Design review of the part built by this model. Coordinates are the model's own, in mm. Face numbers are marked on the shaded views. Give positions to 0.01 mm unless a question says otherwise; leave off trailing zeros. Write each loop counter-clockwise with the first axis right and the second up, starting at its lowest first coordinate (ties: lowest second). Pieces come first, ordered by that corner, then holes. Notation, with made-up numbers: (-32.75, 86.5) -> (-27.75, 86.5) arc R15 cw to (-27.75, 100.5) -> close; hole circle Ø8 at (2.25, -40). An arc over 180 degrees is marked (long way). Use CSV: the item, a comma, the result in double quotes.
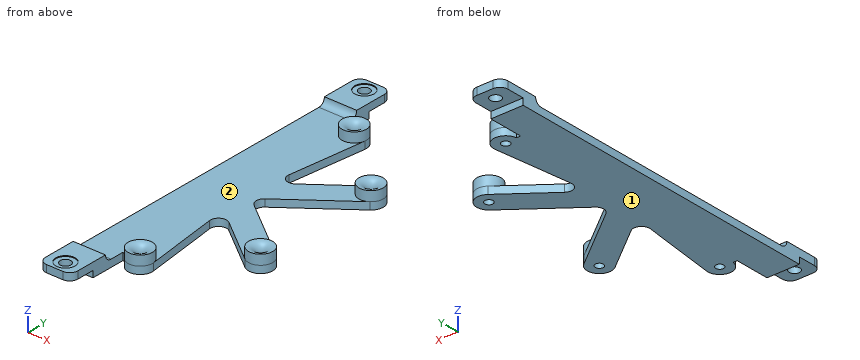
```python
from build123d import *

# Parameters (mm, degrees)
SKETCH_1_W                   = 20
SKETCH_1_H                   = 232
EXTRUDE_1_DEPTH              = 4.5
EXTRUDE_3_DEPTH              = 4.5
FILLET_2_R                   = 4.999999999999999
HOLE_WIZARD_M6_1_D           = 5
FILLET_4_R                   = 4.999999999999999
EXTRUDE_START                = 4
EXTRUDE_4_DEPTH              = 4
SKETCH_9_W                   = 319.0213755361433
SKETCH_9_H                   = 251.11270465686212
CUT_EXTRUDE_1_DEPTH          = 4
FILLET_5_R                   = 4
HOLE_WIZARD_M6_2_D           = 6.6
HOLE_WIZARD_M6_2_CBORE_D     = 12
HOLE_WIZARD_M6_2_CBORE_DEPTH = 0.5
EXTRUDE_START_2              = 6
SKETCH_13_R                  = 2.4999999999999987
SKETCH_13_R_2                = 2.499999999999995
EXTRUDE_5_DEPTH              = 6
FILLET_6_R                   = 5


# Some blends are built 0.0001 mm under size
with BuildPart() as part:
    # 草图1 → 凸台-拉伸1 (new body)
    with BuildSketch(Plane.XY):
        Rectangle(SKETCH_1_W, SKETCH_1_H)
    extrude(amount=EXTRUDE_1_DEPTH)

    # 草图4 → 凸台-拉伸3 (add)
    with BuildSketch(Plane.XY.offset(4.5)):
        with BuildLine():
            Line((67.04532411447143, -34.03426209975627), (22.3753551085413, -8.9e-16))
            Line((22.375355108541303, -2.66e-15), (67.04532411447141, 34.0342620997563))
            ThreePointArc((67.04532411447141, 34.03426209975629), (68.46573790024371, 44.54532411447144), (57.954675885528566, 45.96573790024377))
            Line((57.954675885528566, 45.96573790024377), (19.735945661830147, 16.846705348854464))
            Line((19.73594566183015, 16.846705348854464), (27.438333999755184, 76.54021496777352))
            ThreePointArc((27.438333999755184, 76.54021496777352), (20.959785032226467, 84.9383339997552), (12.561666000244795, 78.45978503222648))
            Line((12.561666000244797, 78.45978503222648), (10.000000000000002, 78.45978503222645))
            Line((10.000000000000002, 78.45978503222645), (9.999999999999897, 58.60687353032759))
            Line((9.999999999999785, 58.606873530327604), (2.561666000244813, 0.9597850322264776))
            ThreePointArc((2.5616660002448137, 0.9597850322264744), (2.5000000000000036, -1.321e-14), (2.561666000244818, -0.9597850322265004))
            Line((2.561666000244811, -0.959785032226501), (9.999999999999945, -58.606873530328755))
            Line((9.999999999999973, -58.606873530328755), (10.000000000000002, -78.45978503222648))
            Line((10.000000000000002, -78.45978503222648), (12.561666000244813, -78.45978503222648))
            ThreePointArc((12.561666000244813, -78.45978503222648), (20.95978503222648, -84.9383339997552), (27.43833399975519, -76.54021496777352))
            Line((27.438333999755194, -76.54021496777352), (19.735945661830147, -16.846705348854485))
            Line((19.735945661830144, -16.84670534885448), (57.95467588552857, -45.96573790024377))
            ThreePointArc((57.95467588552857, -45.96573790024377), (68.46573790024374, -44.54532411447145), (67.04532411447143, -34.034262099756276))
        make_face()
    extrude(amount=-EXTRUDE_3_DEPTH)

    # 圆角2
    fillet_2_edges = [part.edges().sort_by_distance(p)[0] for p in [
        (19.735945661830144, -16.846705348854485, 2.25),
        (22.3753551085413, -1.78e-15, 2.25),
        (19.73594566183015, 16.846705348854464, 2.25),
    ]]
    fillet(fillet_2_edges, radius=FILLET_2_R)

    # Hole Wizard M6 _1 (through all)
    with Locations(Plane.XY.offset(4.5)):
        with Locations((20, 77.5), (62.5, 40), (20, -77.5), (62.5, -40)):
            Hole(HOLE_WIZARD_M6_1_D / 2)

    # 圆角4
    fillet_4_edges = [part.edges().sort_by_distance(p)[0] for p in [
        (10.000000000000002, -116.00000000000001, 2.25),
        (-9.999999999999998, -116.00000000000001, 2.25),
        (-9.999999999999998, 115.99999999999999, 2.25),
        (10.000000000000002, 115.99999999999999, 2.25),
    ]]
    fillet(fillet_4_edges, radius=FILLET_4_R)

    # 草图8 → 凸台-拉伸4 (add)
    with BuildSketch(Plane.XY.offset(4.5).offset(EXTRUDE_START)):
        with BuildLine():
            Line((10, -91), (-10, -91))
            Line((-9.999999999999998, -91.00000000000001), (-9.999999999999998, -111.00000000000001))
            ThreePointArc((-10, -111.00000000000001), (-8.535533905932738, -114.53553390593275), (-5, -116.00000000000001))
            Line((-5, -116.00000000000001), (5.0000000000000036, -116.00000000000001))
            ThreePointArc((5.000000000000003, -116.00000000000001), (8.535533905932741, -114.53553390593275), (10.000000000000004, -111.00000000000001))
            Line((10.000000000000005, -111.00000000000001), (10.000000000000004, -91))
        make_face()
        with BuildLine():
            Line((-9.999999999999998, 110.99999999999993), (-9.999999999999998, 91))
            Line((-10, 91), (10, 91))
            Line((10.000000000000002, 91), (10.000000000000002, 110.99999999999993))
            ThreePointArc((10, 110.99999999999993), (8.535533905932763, 114.53553390593271), (5.000000000000003, 115.99999999999999))
            Line((5.000000000000003, 115.99999999999999), (-4.999999999999999, 115.99999999999999))
            ThreePointArc((-4.999999999999999, 115.99999999999999), (-8.535533905932759, 114.53553390593271), (-9.999999999999996, 110.99999999999993))
        make_face()
    extrude(amount=-EXTRUDE_4_DEPTH)

    # 草图9 → 切除-拉伸1 (cut)
    with BuildSketch(Plane(origin=(0, 0, 0), x_dir=(-1, 0, 0), z_dir=(0, 0, -1))):
        Rectangle(SKETCH_9_W, SKETCH_9_H)
        Polygon((-82.97210234114478, 100), (82.97210234114469, 100), (82.97210234114472, -100), (-82.97210234114475, -100), align=None, mode=Mode.SUBTRACT)
    extrude(amount=-CUT_EXTRUDE_1_DEPTH, mode=Mode.SUBTRACT)

    # 圆角5
    fillet_5_edges = [part.edges().sort_by_distance(p)[0] for p in [
        (0, -91, 4.5),
        (0, 91, 4.5),
    ]]
    fillet(fillet_5_edges, radius=FILLET_5_R - 0.0001)  # a hair under: the kernel refuses the full size

    # M6 六角头螺栓的柱形沉头孔2 (through all)
    with Locations(Plane.XY.offset(8.5)):
        with Locations((0, 108.25), (0, -108.25)):
            CounterBoreHole(HOLE_WIZARD_M6_2_D / 2, HOLE_WIZARD_M6_2_CBORE_D / 2, HOLE_WIZARD_M6_2_CBORE_DEPTH)

    # 草图13 → 凸台-拉伸5 (add)
    # profile 1 of 4: a face of its own
    with BuildSketch(Plane.XY.offset(4.5).offset(EXTRUDE_START_2)):
        with BuildLine():
            ThreePointArc((27.438333999755173, 76.54021496777352), (27.484567622720885, 77.01911799688693), (27.499999999999986, 77.5))
            ThreePointArc((27.499999999999986, 77.5), (20.480882003113063, 84.9845676227209), (12.561666000244797, 78.45978503222648))
            ThreePointArc((12.561666000244797, 78.45978503222648), (19.040214967773508, 70.06166600024481), (27.438333999755173, 76.54021496777352))
        make_face()
        with Locations((19.999999999999986, 77.5)):
            Circle(SKETCH_13_R, mode=Mode.SUBTRACT)
    # profile 2 of 4: a face of its own
    with BuildSketch(Plane.XY.offset(4.5).offset(EXTRUDE_START_2)):
        with BuildLine():
            ThreePointArc((70, 40.00000000000002), (65.82866858829955, 46.72086046792137), (57.954675885528566, 45.96573790024377))
            ThreePointArc((57.954675885528566, 45.96573790024377), (56.53426209975625, 35.454675885528594), (67.04532411447143, 34.034262099756276))
            ThreePointArc((67.04532411447143, 34.034262099756276), (69.22086046792134, 36.671331411700464), (70, 40.00000000000002))
        make_face()
        with Locations((62.49999999999999, 40.00000000000002)):
            Circle(SKETCH_13_R_2, mode=Mode.SUBTRACT)
    # profile 3 of 4: a face of its own
    with BuildSketch(Plane.XY.offset(4.5).offset(EXTRUDE_START_2)):
        with BuildLine():
            ThreePointArc((69.99999999999999, -40.00000000000002), (69.22086046792133, -36.67133141170047), (67.04532411447141, -34.03426209975629))
            ThreePointArc((67.04532411447141, -34.03426209975629), (56.53426209975626, -35.4546758855286), (57.95467588552858, -45.96573790024376))
            ThreePointArc((57.95467588552858, -45.96573790024376), (65.82866858829955, -46.720860467921355), (69.99999999999999, -40.00000000000002))
        make_face()
        with Locations((62.49999999999999, -40.00000000000002)):
            Circle(SKETCH_13_R_2, mode=Mode.SUBTRACT)
    # profile 4 of 4: a face of its own
    with BuildSketch(Plane.XY.offset(4.5).offset(EXTRUDE_START_2)):
        with BuildLine():
            ThreePointArc((27.438333999755177, -76.54021496777352), (19.040214967773533, -70.06166600024483), (12.561666000244838, -78.45978503222648))
            ThreePointArc((12.561666000244838, -78.45978503222648), (20.48088200311308, -84.98456762272087), (27.499999999999986, -77.5))
            ThreePointArc((27.499999999999986, -77.5), (27.484567622720885, -77.01911799688692), (27.438333999755177, -76.54021496777352))
        make_face()
        with Locations((20.000000000000007, -77.5)):
            Circle(SKETCH_13_R, mode=Mode.SUBTRACT)
    extrude(amount=-EXTRUDE_5_DEPTH)

    # 圆角6
    # the kernel refuses this fillet: 5 mm, written as the material it takes off along each edge
    with BuildSketch(Plane(origin=(19.999999999999986, 77.5, 10.5), x_dir=(1, 0, 0), z_dir=(0, -1, 0))) as fillet_6_piece_1:
        with BuildLine():
            CenterArc((2.5 + FILLET_6_R, -FILLET_6_R), FILLET_6_R, 90.00000000000017, 89.99999999999983)
            Line((2.5 + FILLET_6_R, 0), (2.5, 0))
            Line((2.5, 0), (2.500000000000014, -FILLET_6_R))
        make_face()
    revolve(axis=Axis((19.999999999999986, 77.5, 10.5), (0, 0, 1)), mode=Mode.SUBTRACT)
    with BuildSketch(Plane(origin=(62.49999999999999, 40.00000000000002, 10.5), x_dir=(1, 0, 0), z_dir=(0, -1, 0))) as fillet_6_piece_2:
        with BuildLine():
            CenterArc((2.499999999999993 + FILLET_6_R, -FILLET_6_R), FILLET_6_R, 90.00000000000017, 89.99999999999983)
            Line((2.499999999999993 + FILLET_6_R, 0), (2.499999999999993, 0))
            Line((2.499999999999993, 0), (2.500000000000007, -FILLET_6_R))
        make_face()
    revolve(axis=Axis((62.49999999999999, 40.00000000000002, 10.5), (0, 0, 1)), mode=Mode.SUBTRACT)
    with BuildSketch(Plane(origin=(62.49999999999999, -40.00000000000002, 10.5), x_dir=(1, 0, 0), z_dir=(0, -1, 0))) as fillet_6_piece_3:
        with BuildLine():
            CenterArc((2.499999999999993 + FILLET_6_R, -FILLET_6_R), FILLET_6_R, 90.00000000000017, 89.99999999999983)
            Line((2.499999999999993 + FILLET_6_R, 0), (2.499999999999993, 0))
            Line((2.499999999999993, 0), (2.500000000000007, -FILLET_6_R))
        make_face()
    revolve(axis=Axis((62.49999999999999, -40.00000000000002, 10.5), (0, 0, 1)), mode=Mode.SUBTRACT)
    with BuildSketch(Plane(origin=(20.000000000000007, -77.5, 10.5), x_dir=(1, 0, 0), z_dir=(0, -1, 0))) as fillet_6_piece_4:
        with BuildLine():
            CenterArc((2.5 + FILLET_6_R, -FILLET_6_R), FILLET_6_R, 89.99999999999993, 90.00000000000006)
            Line((2.5 + FILLET_6_R, 0), (2.5, 0))
            Line((2.5, 0), (2.499999999999993, -FILLET_6_R))
        make_face()
    revolve(axis=Axis((20.000000000000007, -77.5, 10.5), (0, 0, 1)), mode=Mode.SUBTRACT)


solid = part.part
```
(1) Take a section at C-C (x = 62.5). Write out the cut boundary in (y, z).
Established:
outline,"(-47.5, 0) -> (-42.5, 0) -> (-42.5, 5.5) arc R5 ccw to (-47.5, 10.5) -> close; (-37.5, 0) -> (-30.57, 0) -> (-30.57, 4.5) -> (-32.5, 4.5) -> (-32.5, 10.5) arc R5 ccw to (-37.5, 5.5) -> close; (30.57, 0) -> (37.5, 0) -> (37.5, 5.5) arc R5 ccw to (32.5, 10.5) -> (32.5, 4.5) -> (30.57, 4.5) -> close; (42.5, 0) -> (47.5, 0) -> (47.5, 10.5) arc R5 ccw to (42.5, 5.5) -> close"
(2) For line 1 along Y through (x, z) = (62.5, 5.75); line 2 along Y through (x, z) = (20, 1.7); line 3 along X through (y, z) = (77.5, 4.9), list the stretches that pass through material, from the lowest coordinate up. Write a range as [from, to].
Established:
line 1,"y = [-47.5, -42.51], [-37.49, -32.5], [32.5, 37.49], [42.51, 47.5]"
line 2,"y = [-85, -80], [-75, 75], [80, 85]"
line 3,"x = [12.5, 17.5], [22.5, 27.5]"
(3) Take a section at A-A (y = -108.25). Write out the cut boundary in (x, z).
Established:
outline,"(-10, 4) -> (-3.3, 4) -> (-3.3, 8) -> (-6, 8) -> (-6, 8.5) -> (-10, 8.5) -> close; (3.3, 4) -> (10, 4) -> (10, 8.5) -> (6, 8.5) -> (6, 8) -> (3.3, 8) -> close"
(4) Take a section at B-B (x = 0). State how many separate pieces and enclosed holes the cut face has, then the cut area to 3 significant figures.
Established:
separate pieces,"3"
enclosed holes,"0"
area,"1,060 mm2"
(5) Clearance check with flat-ended pins moving along their axes: pin 1 (9.5 mm diameter, centred on x = 2, y = 107, fed in from +Z); pin 2 (17.5 mm diameter, centred on x = -2, y = -108.5, fed in from -Z); pin 3 (3 mm diameter, centred on y = -92, z = 6, fed in from +X); pin 4 (6 mm diameter, centred on x = 2.5, y = -108.5, fed in from +Z). State where each tip first meets the part, or that it passes through.
Established:
pin 1,"stops at z = 8.5"
pin 2,"stops at z = 0"
pin 3,"stops at x = 10"
pin 4,"stops at z = 8"
(6) Take a section at D-D (x = 49). Write out the cut boundary in (y, z), then the cut area to 3 significant figures.
Established:
outline,"(-39.14, 0) -> (-20.29, 0) -> (-20.29, 4.5) -> (-39.14, 4.5) -> close; (20.29, 0) -> (39.14, 0) -> (39.14, 4.5) -> (20.29, 4.5) -> close"
area,"170 mm2"
(7) Mouldability with a two-part tool opening along Y and no side actions: class the marked faces 1 and 2 as +Y half, -Y half, draft (parallel to the pull), parting line (faces both ways), or undercut.
Established:
face 1,"draft"
face 2,"undercut"
